The listing builds one solid part. Answer for the finished solid, in the listing's coordinates (mm). Face numbers are marked on the shaded views. A direction names the side the tool comes from. Round coordinates to 2 decimals unless told otherwise and drop trailing zeros. Write each loop counter-clockwise with the first axis right and the second up, starting at its lowest first coordinate (ties: lowest second). Pieces come first, ordered by that corner, then holes.
(1) A cutting plane is placed at C-C, the plane y = 6.5. Give the number of separate pieces and of enclosed holes in the cut face, and give its area (3 significant figures).
(2) Find the intervals of material crossed by probe 1 along X at (y, z) = (3.25, 50); probe 2 along X at (y, z) = (9.5, 67); probe 3 along Z at (x, y) = (38, 3.8), in increasing order.
(3) A cutting plane is placed at A-A, the plane z = 50. Give the vertices of the cut face in (x, y), and give its area (3 significant figures).
(4) For the marked faces 1, 2 and 3, determine the directions among +Z, -Z, +X, -X, +Y, -Y from which every point of the face is accessible in a straight line to the end or side of a thin tool.
(5) A cutting plane is placed at B-B, the plane x = -31. Give the vertices of the cut face in (y, z), and give its area (3 significant figures).
(6) Each of these flat-tipped pins is pushed along its axis until it touches: pin 1 Ø5 at (x, y) = (27.5, 5) entering from +Z; pin 2 Ø3 at (x, y) = (-36, 4) entering from +Z; pin 3 Ø3.5 at (x, y) = (-15, 6.5) entering from +Z; pin 4 Ø4.5 at (x, z) = (38, 50) entering from -Y. Where does it stop, or does it pass through?
(7) The mould has two halves that part along X. Classify the marked faces 4, 5 and 6: +X half, -X half, draft (parallel to the pull), parting line (faces both ways), or undercut.
from build123d import *

# Parameters (mm, degrees)
ESQUISSE2_R             = 2.5
BOSS_EXTRU_1_DEPTH      = 10
CONG_1_R                = 3
ESQUISSE4_R             = 1.25
ENL_V_MAT_EXTRU_2_DEPTH = 109.719823399
ENL_V_MAT_EXTRU_3_DEPTH = 5


with BuildPart() as part:
    # Esquisse2 → Boss.-Extru.1 (new body)
    with BuildSketch(Plane(origin=(0, 0, 0), x_dir=(1, 0, 0), z_dir=(0, 1, 0))):
        with BuildLine():
            Line((0, -98), (-3.514709064, -98))
            ThreePointArc((-3.514709064, -98), (-6.748469646, -92.676394089), (-10.808475025, -87.952588026))
            ThreePointArc((-10.808475025, -87.952588026), (-12.561008366, -85.888384873), (-13.92457187, -83.548939995))
            Line((-13.92457187, -83.548939995), (-25, -60))
            Line((-25, -60), (-46, -60))
            Line((-46, -60), (-46, -30))
            Line((-46, -30), (0, -30))
            Line((0, -30), (0, -43.5))
            Line((0, -43.5), (0, -46.5))
            Line((0, -46.5), (0, -65))
            ThreePointArc((0, -65), (-12, -77), (0, -89))
            Line((0, -89), (0, -98))
        make_face()
        with Locations(Location((-38, -50, 0), (0, 0, 270))):
            Circle(ESQUISSE2_R, mode=Mode.SUBTRACT)
    extrude(amount=BOSS_EXTRU_1_DEPTH)

    # Congé1
    cong_1_edges = [part.edges().sort_by_distance(p)[0] for p in [
        (-46, 5, 30),
        (-3.514709064, 5, 98),
        (-25, 5, 60),
        (-46, 5, 60),
    ]]
    fillet(cong_1_edges, radius=CONG_1_R)

    # Symétrie1: part across face


with BuildPart() as part_1:
    add(part.part)
    add(part.part.mirror(Plane(origin=(0, 5, 47.5), x_dir=(0, 0, 1), z_dir=(1, 0, 0))))

    # Esquisse4 → Enlèv. mat.-Extru.2 (cut, through all)
    with BuildSketch(Plane(origin=(0, 10, 0), x_dir=(1, 0, 0), z_dir=(0, 1, 0))):
        with Locations(Location((-14.526993136, -68.170137576, 0), (0, 0, 270))):
            Circle(ESQUISSE4_R)
        with Locations(Location((0, -94, 0), (0, 0, 270))):
            Circle(ESQUISSE4_R)
        with Locations(Location((14.526993136, -68.170137576, 0), (0, 0, 90))):
            Circle(ESQUISSE4_R)
    extrude(amount=-ENL_V_MAT_EXTRU_2_DEPTH, mode=Mode.SUBTRACT)

    # Esquisse5 → Enlèv. mat.-Extru.3 (cut)
    with BuildSketch(Plane(origin=(0, 10, 0), x_dir=(1, 0, 0), z_dir=(0, 1, 0))):
        Polygon((-11.351566655, -68.170137576), (-12.939279895, -65.420137576), (-16.114706376, -65.420137576), (-17.702419616, -68.170137576), (-16.114706376, -70.920137576), (-12.939279895, -70.920137576), align=None)
        Polygon((17.702419616, -68.170137576), (16.114706376, -65.420137576), (12.939279895, -65.420137576), (11.351566655, -68.170137576), (12.939279895, -70.920137576), (16.114706376, -70.920137576), align=None)
        Polygon((3.175426481, -94), (1.58771324, -91.25), (-1.58771324, -91.25), (-3.175426481, -94), (-1.58771324, -96.75), (1.58771324, -96.75), align=None)
        Polygon((-34, -47.690598923), (-38, -45.381197846), (-42, -47.690598923), (-42, -52.309401077), (-38, -54.618802154), (-34, -52.309401077), align=None)
        Polygon((42, -52.309401077), (42, -47.690598923), (38, -45.381197846), (34, -47.690598923), (34, -52.309401077), (38, -54.618802154), align=None)
    extrude(amount=-ENL_V_MAT_EXTRU_3_DEPTH, mode=Mode.SUBTRACT)


solid = part_1.part
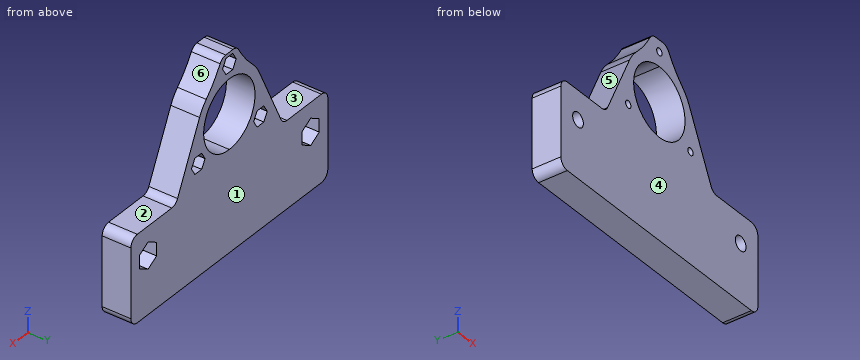
Solutions:
1. separate pieces: 1
1. enclosed holes: 6
1. area: 3,270 mm2
2. probe 1: x = -46 to -40.5, -35.5 to 35.5, 40.5 to 46
2. probe 2: x = -21.71 to -17.03, -12.03 to -6.63, 6.63 to 12.03, 17.03 to 21.71
2. probe 3: z = 30 to 47.5, 52.5 to 60
3. outline: (-46, 0) - (-40.5, 0) - (-40.5, 5) - (-42, 5) - (-42, 10) - (-46, 10) - close; (-35.5, 0) - (35.5, 0) - (35.5, 5) - (34, 5) - (34, 10) - (-34, 10) - (-34, 5) - (-35.5, 5) - close; (40.5, 0) - (46, 0) - (46, 10) - (42, 10) - (42, 5) - (40.5, 5) - close
3. area: 790 mm2
4. face 1: +Z, -Z, +X, -X, +Y
4. face 2: +Z, +X, +Y, -Y
4. face 3: +Z, -X, +Y, -Y
5. outline: (0, 30) - (10, 30) - (10, 60) - (0, 60) - close
5. area: 300 mm2
6. pin 1: stops at z = 60.68
6. pin 2: stops at z = 60
6. pin 3: stops at z = 84.82
6. pin 4: passes through
7. face 4: draft
7. face 5: -X half
7. face 6: +X half
